Can you work these out from the model? Positions are in its coordinate system, mm. A direction names the side the tool comes from. Round coordinates to 2 decimals unless told otherwise and drop trailing zeros. Order: outer loops, then holes, each group sorted by start corner. A loop starts at its lowest first (then second) coordinate and runs counter-clockwise, first axis right, second up.
Q1. If we section it at A-A (z = 4): Please give me the cut outline in (x, y).
Q2. If I drill on line 1 (X direction, y = 1.4, z = 4); line 2 (Y direction, x = -11, z = -5); line 3 (Z direction, x = 11.5, y = 2.95), over which ranges is the centre line in solid material (lowest first)?
Q3. We'd pull the mould along X, two halves only. Please class faces 1 (the face through (4.541, 1.521, 5.717)), 2 (the face through (-9, 3, -14)), 3 (the face through (-1.2, 1.7, -13.9)): pulls with the +X half, pulls with the -X half, needs draft (parallel to the pull), parting line crosses it, or undercut.
Q4. If we section it at C-C (x = 4): Please give me the cut outline in (y, z).
Q5. Will these pins go through, and if not, where does the flat tip stop? P1, Ø4, axis at x = -11, z = -16, coming from the -Y side; P2, Ø3, axis at y = 3.5, z = -12, coming from the +X side; P3, Ø1.5, axis at y = 1.5, z = 4, coming from the +X side; P4, Ø3, axis at x = 15.5, y = 1.5, coming from the +Z side.
Q6. If we section it at B-B (y = 2.4): Please give me the cut outline in (x, z).
Q7. For faces 4 (the face through (12, 3, -8)), 5 (the face through (-14.43, 4.27, -23.4)), which set-ups out of +Z, -Z, +X, -X, +Y, -Y let a thin tool reach every point of the face, with its end or its side?
from build123d import *

# Parameters (mm, degrees)
SKETCH1_W           = 20
SKETCH1_H           = 24
BOSS_EXTRUDE1_DEPTH = 3
SKETCH2_W           = 8
SKETCH2_H           = 8
SKETCH2_R           = 1.8
BOSS_EXTRUDE2_DEPTH = 3
FILLET1_R           = 2
CHAMFER1_SIZE       = 2
SKETCH3_W           = 18
SKETCH3_H           = 24
BOSS_EXTRUDE3_DEPTH = 2.5
CHAMFER2_SIZE       = 2.5
CUT_EXTRUDE4_DEPTH  = 4
FILLET2_R           = 2
CUT_EXTRUDE3_DEPTH  = 0.4


with BuildPart() as part:
    # Sketch1 → Boss-Extrude1 (new body)
    with BuildSketch(Plane(origin=(0, 0, 0), x_dir=(1, 0, 0), z_dir=(0, 1, 0))):
        with Locations((10, 12)):
            Rectangle(SKETCH1_W, SKETCH1_H)
    extrude(amount=BOSS_EXTRUDE1_DEPTH)

    # Sketch2 → Boss-Extrude2 (add)
    with BuildSketch(Plane(origin=(0, 3, 0), x_dir=(1, 0, 0), z_dir=(0, 1, 0))):
        with Locations((4, -4)):
            Rectangle(SKETCH2_W, SKETCH2_H)
        with Locations(Location((4, -4, 0), (0, 0, 270))):
            Circle(SKETCH2_R, mode=Mode.SUBTRACT)
    extrude(amount=-BOSS_EXTRUDE2_DEPTH)

    # Fillet1
    fillet1_edges = [part.edges().sort_by_distance(p)[0] for p in [
        (8, 1.5, 0),
        (8, 1.5, 8),
        (0, 1.5, 8),
    ]]
    fillet(fillet1_edges, radius=FILLET1_R)

    # Chamfer1
    chamfer1_edges = [part.edges().sort_by_distance(p)[0] for p in [
        (20, 1.5, 0),
    ]]
    chamfer(chamfer1_edges, length=CHAMFER1_SIZE)

    # Sketch3 → Boss-Extrude3 (add)
    with BuildSketch(Plane(origin=(0, 3, 0), x_dir=(1, 0, 0), z_dir=(0, 1, 0))):
        with Locations((-6, 12)):
            Rectangle(SKETCH3_W, SKETCH3_H)
    extrude(amount=BOSS_EXTRUDE3_DEPTH)

    # Chamfer2
    chamfer2_edges = [part.edges().sort_by_distance(p)[0] for p in [
        (0, 3, -12),
        (3, 3, -12),
    ]]
    chamfer(chamfer2_edges, length=CHAMFER2_SIZE - 0.0001)  # a hair under: the kernel refuses the full size

    # Sketch5 → Cut-Extrude4 (cut)
    with BuildSketch(Plane.XY):
        Polygon((-15, 3), (-2.5, 3), (0, 0.5), (0, 3), (5.5, 3), (3, 5.5), (-15, 5.5), align=None)
    extrude(amount=-CUT_EXTRUDE4_DEPTH, mode=Mode.SUBTRACT)

    # Fillet2
    fillet2_edges = [part.edges().sort_by_distance(p)[0] for p in [
        (-15, 4.25, -24),
        (-15, 4.25, -4),
    ]]
    fillet(fillet2_edges, radius=FILLET2_R)

    # Sketch4 → Cut-Extrude3 (cut)
    with BuildSketch(Plane.XZ):
        Polygon((8, 2), (8, 0), (0, 0), (0, -24), (20, -24), (20, 0), (20, 2), align=None)
    extrude(amount=-CUT_EXTRUDE3_DEPTH, mode=Mode.SUBTRACT)


solid = part.part
Solution:
1. outline: (0, 0) - (2.2, 0) - (2.2, 3) - (0, 3) - close; (5.8, 0) - (8, 0) - (8, 3) - (5.8, 3) - close
2. line 1: x = 0 to 2.2, 5.8 to 8
2. line 2: y = 3 to 5.5
2. line 3: z = -24 to 0
3. face 1: undercut
3. face 2: needs draft
3. face 3: pulls with the -X half
4. outline: (0, 0) - (0.4, 0) - (0.4, -24) - (4.5, -24) - (4.5, -4) - (3, -4) - (3, 2.2) - (0, 2.2) - close; (0, 5.8) - (3, 5.8) - (3, 8) - (0, 8) - close
5. P1: stops at y = 3
5. P2: stops at x = 20
5. P3: stops at x = 8
5. P4: stops at z = 0
6. outline: (-1.9, -24) - (20, -24) - (20, -2) - (18, 0) - (10, 0) arc R2 cw to (8, 2) - (8, 6) arc R2 ccw to (6, 8) - (2, 8) arc R2 ccw to (0, 6) - (0, -4) - (-1.9, -4) - close; hole circle Ø3.6 at (4, 4)
7. face 4: +Z, +X, +Y
7. face 5: -Z, -X, +Y, -Y
